The figure shows three views and two pictorial views of one solid part (mm, origin at its lowest corner). Answer the questions. A direction names the side the tool comes from. Give positions to 0.01 mm unless a question says otherwise; leave off trailing zeros. Loops run counter-clockwise (first coordinate to the right, second up) from the corner with the lowest first, then second, coordinate; pieces in that order, holes last. Notation, with made-up numbers: (54.5, 50.5) -> (61.5, 50.5) arc R18 cw to (61.5, 75.5) -> close; hole circle Ø4 at (-34, -5.75). An arc over 180 degrees is marked (long way). Answer as CSV lines item,"result". Start each with the question number.
1. Find section A-A, the plane z = 7.5. Give the vertices of the cut face in (x, y).
2. Find section C-C, the plane x = 10.5. Give the vertices of the cut face in (y, z).
3. Find section B-B, the plane y = 119.5. Give the vertices of the cut face in (x, z).
4. Find the intervals of material crossed by line 1 along X through (y, z) = (89, 8); line 2 along Y through (x, z) = (29, 10.25); line 3 along X through (y, z) = (79, 6.5), in increasing order.
5. A tool of negligible diameter and unlimited length cuts with its end or side. For the marked faces 1 and 2, from which of +Z, -Z, +X, -X, +Y, -Y can it reach the whole face along a straight path? Write none if from no direction.
6. Flat-ended cylindrical pins translate along their axes: pin 1 Ø8 at (x, y) = (11.5, 188) entering from -Z; pin 2 Ø10 at (x, y) = (22.5, 138) entering from +Z; pin 3 Ø3 at (x, y) = (14.5, 205.5) entering from +Z. Find the tip coordinate at first contact, or state that the pin passes through.
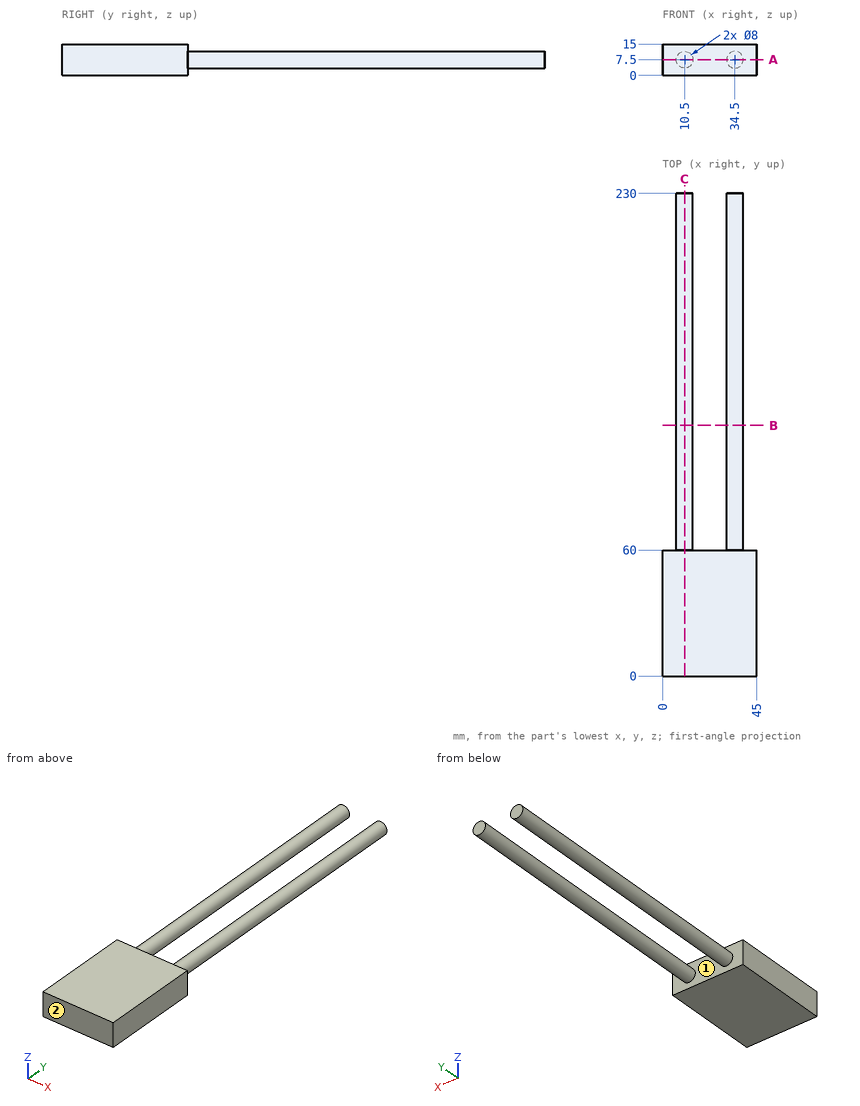
Resolved:
1,outline,"(0, 0) -> (45, 0) -> (45, 60) -> (38.5, 60) -> (38.5, 230) -> (30.5, 230) -> (30.5, 60) -> (14.5, 60) -> (14.5, 230) -> (6.5, 230) -> (6.5, 60) -> (0, 60) -> close"
2,outline,"(0, 0) -> (60, 0) -> (60, 3.5) -> (230, 3.5) -> (230, 11.5) -> (60, 11.5) -> (60, 15) -> (0, 15) -> close"
3,outline,"circle Ø8 at (10.5, 7.5); circle Ø8 at (34.5, 7.5)"
4,line 1,"x = 6.53 to 14.47, 30.53 to 38.47"
4,line 2,"y = 0 to 60"
4,line 3,"x = 6.63 to 14.37, 30.63 to 38.37"
5,face 1,"+Y"
5,face 2,"+Z, -Z, +X, -X, -Y"
6,pin 1,"stops at z = 3.5"
6,pin 2,"passes through"
6,pin 3,"stops at z = 10.62"
